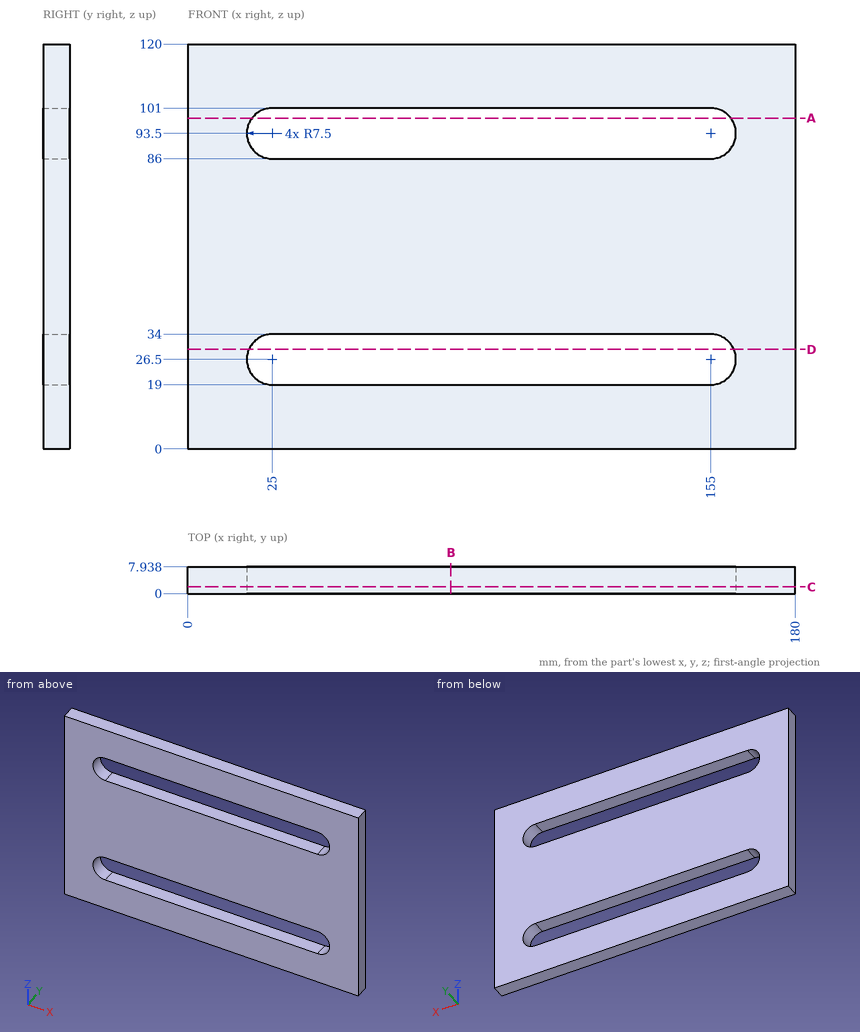
Input: dimensioned drawing with shaded views. Units: mm. Origin: part minimum x, y, z. Coordinates: 2 decimals unless noted, no trailing zeros. Write each loop counter-clockwise with the first axis right and the second up, starting at its lowest first coordinate (ties: lowest second). Pieces come first, ordered by that corner, then holes. Notation, with made-up numbers: M -2,27 L 41,27 A24 ccw 41,45 Z; hole C 70,13 d2. An arc over 180 degrees is marked long. Answer as CSV lines item,"result". Start each with the question number.
Q1. Cut plane A-A on z = 98. Return the cut outline in (x, y).
Q2. Pin query (flat end, axial travel): P1, Ø1, axis at x = 135, z = 60.5, coming from the -Y side. Return the tip coordinate at first contact, or that it passes through.
Q3. Cut plane B-B on x = 78. Return the cut outline in (y, z).
Q4. Cut plane D-D on z = 29.5. Return the cut outline in (x, y), then the cut area to 3 significant figures.
Q5. Cut plane C-C on y = 2. Return the cut outline in (x, z).
Q6. Line query: line 1 (Z direction, x = 135, y = 5.75); line 2 (X direction, y = 2.25, z = 26); line 3 (X direction, y = 6, z = 33) (1 decimal). Output: solid intervals per line, ascending. Write a range as from..to.
Findings below:
1,outline,"M 0,0 L 19,0 L 19,7.94 L 0,7.94 Z; M 161,0 L 180,0 L 180,7.94 L 161,7.94 Z"
2,P1,"stops at y = 0"
3,outline,"M 0,0 L 7.94,0 L 7.94,19 L 0,19 Z; M 0,34 L 7.94,34 L 7.94,86 L 0,86 Z; M 0,101 L 7.94,101 L 7.94,120 L 0,120 Z"
4,outline,"M 0,0 L 18.13,0 L 18.13,7.94 L 0,7.94 Z; M 161.87,0 L 180,0 L 180,7.94 L 161.87,7.94 Z"
4,area,"288 mm2"
5,outline,"M 0,0 L 180,0 L 180,120 L 0,120 Z; hole M 25,19 L 155,19 A7.5 ccw 155,34 L 25,34 A7.5 ccw Z; hole M 25,86 L 155,86 A7.5 ccw 155,101 L 25,101 A7.5 ccw Z"
6,line 1,"z = 0..19, 34..86, 101..120"
6,line 2,"x = 0..17.52, 162.48..180"
6,line 3,"x = 0..21.3, 158.7..180"
